```python
from build123d import *

# Parameters (mm, degrees)
F1_DEPTH = 6
F2_R     = 1
F3_R     = 10
F4_DEPTH = 16
F6_DEPTH = 25


with BuildPart() as f1:
    # F0 (on Front) → F1 (new body)
    with BuildSketch(Plane.XZ):
        with BuildLine():
            Line((0.9983844832, 7.6002832444), (-0.5016155168, 7.6002832444))
            ThreePointArc((-0.5016155168, 7.6002832444), (-2.6229358604, 6.7216035879), (-3.5016155168, 4.6002832444))
            Line((-3.5016155168, 4.6002832444), (-3.5016155168, 1.6002832444))
            ThreePointArc((-3.5016155168, 1.6002832444), (-2.6229358604, -0.5210370992), (-0.5016155168, -1.3997167556))
            Line((-0.5016155168, -1.3997167556), (0.9983844832, -1.3997167556))
            ThreePointArc((0.9983844832, -1.3997167556), (3.4732582173, -0.3745904898), (4.4983844832, 2.1002832444))
            Line((4.4983844832, 2.1002832444), (4.4983844832, 4.1002832444))
            ThreePointArc((4.4983844832, 4.1002832444), (3.4732582173, 6.5751569785), (0.9983844832, 7.6002832444))
        make_face()
    extrude(amount=F1_DEPTH)

    # F2
    f2_edges = [f1.edges().sort_by_distance(p)[0] for p in [
        (3.473258, -6, 6.575157),
        (0.248384, -6, 7.600283),
        (-2.622936, -6, 6.721604),
        (-3.501616, -6, 3.100283),
        (-2.622936, -6, -0.521037),
        (0.248384, -6, -1.399717),
        (3.473258, -6, -0.37459),
        (4.498384, -6, 3.100283),
    ]]
    fillet(f2_edges, radius=F2_R)

    # F3 (on face) → F4 (join)
    with BuildSketch(Plane(origin=(0, 0, 0), x_dir=(-1, 0, 0), z_dir=(0, 1, 0))):
        with Locations((-0.2483844832, 3.1002832444)):
            Circle(F3_R)
        with BuildLine():
            Line((3.5016155168, 4.6002832444), (3.5016155168, 3.1002832444))
            Line((3.5016155168, 3.1002832444), (3.5016155168, 1.6002832444))
            ThreePointArc((3.5016155168, 1.6002832444), (2.6229358604, -0.5210370992), (0.5016155168, -1.3997167556))
            Line((0.5016155168, -1.3997167556), (-0.2483844832, -1.3997167556))
            Line((-0.2483844832, -1.3997167556), (-0.9983844832, -1.3997167556))
            ThreePointArc((-0.9983844832, -1.3997167556), (-3.4732582173, -0.3745904898), (-4.4983844832, 2.1002832444))
            Line((-4.4983844832, 2.1002832444), (-4.4983844832, 3.1002832444))
            Line((-4.4983844832, 3.1002832444), (-4.4983844832, 4.1002832444))
            ThreePointArc((-4.4983844832, 4.1002832444), (-3.4732582173, 6.5751569785), (-0.9983844832, 7.6002832444))
            Line((-0.9983844832, 7.6002832444), (-0.2483844832, 7.6002832444))
            Line((-0.2483844832, 7.6002832444), (0.5016155168, 7.6002832444))
            ThreePointArc((0.5016155168, 7.6002832444), (2.6229358604, 6.7216035879), (3.5016155168, 4.6002832444))
        make_face(mode=Mode.SUBTRACT)
        with BuildLine():
            Line((-0.2483844832, -1.3997167556), (-0.2483844832, 3.1002832444))
            Line((-0.2483844832, 3.1002832444), (-4.4983844832, 3.1002832444))
            Line((-4.4983844832, 3.1002832444), (-4.4983844832, 2.1002832444))
            ThreePointArc((-4.4983844832, 2.1002832444), (-3.4732582173, -0.3745904898), (-0.9983844832, -1.3997167556))
            Line((-0.9983844832, -1.3997167556), (-0.2483844832, -1.3997167556))
        make_face()
        with BuildLine():
            Line((-4.4983844832, 3.1002832444), (-0.2483844832, 3.1002832444))
            Line((-0.2483844832, 3.1002832444), (-0.2483844832, 7.6002832444))
            Line((-0.2483844832, 7.6002832444), (-0.9983844832, 7.6002832444))
            ThreePointArc((-0.9983844832, 7.6002832444), (-3.4732582173, 6.5751569785), (-4.4983844832, 4.1002832444))
            Line((-4.4983844832, 4.1002832444), (-4.4983844832, 3.1002832444))
        make_face()
        with BuildLine():
            Line((3.5016155168, 1.6002832444), (3.5016155168, 3.1002832444))
            Line((3.5016155168, 3.1002832444), (-0.2483844832, 3.1002832444))
            Line((-0.2483844832, 3.1002832444), (-0.2483844832, -1.3997167556))
            Line((-0.2483844832, -1.3997167556), (0.5016155168, -1.3997167556))
            ThreePointArc((0.5016155168, -1.3997167556), (2.6229358604, -0.5210370992), (3.5016155168, 1.6002832444))
        make_face()
        with BuildLine():
            Line((-0.2483844832, 3.1002832444), (3.5016155168, 3.1002832444))
            Line((3.5016155168, 3.1002832444), (3.5016155168, 4.6002832444))
            ThreePointArc((3.5016155168, 4.6002832444), (2.6229358604, 6.7216035879), (0.5016155168, 7.6002832444))
            Line((0.5016155168, 7.6002832444), (-0.2483844832, 7.6002832444))
            Line((-0.2483844832, 7.6002832444), (-0.2483844832, 3.1002832444))
        make_face()
    extrude(amount=F4_DEPTH)

    # F5 (on face) → F6 (cut)
    with BuildSketch(Plane.XZ):
        with BuildLine():
            Line((-0.0016155168, 12.6002832444), (0.2483844832, 12.6002832444))
            Line((0.2483844832, 12.6002832444), (0.2483844832, 13.1002832444))
            ThreePointArc((0.2483844832, 13.1002832444), (0.1233747149, 13.0995018417), (-0.0016155168, 13.0971577559))
            Line((-0.0016155168, 13.0971577559), (-0.0016155168, 12.6002832444))
        make_face()
        with BuildLine():
            Line((0.2483844832, 13.1002832444), (0.2483844832, 12.6002832444))
            Line((0.2483844832, 12.6002832444), (0.4983844832, 12.6002832444))
            Line((0.4983844832, 12.6002832444), (0.4983844832, 13.0971577559))
            ThreePointArc((0.4983844832, 13.0971577559), (0.3733942515, 13.0995018417), (0.2483844832, 13.1002832444))
        make_face()
    extrude(amount=-F6_DEPTH, mode=Mode.SUBTRACT)


solid = f1.part
```
For this review, take the finished solid that the model builds, in its own axes (mm). A direction names the side the tool comes from. Give positions to 0.01 mm unless a question says otherwise; leave off trailing zeros. Write each loop counter-clockwise with the first axis right and the second up, starting at its lowest first coordinate (ties: lowest second). Pieces come first, ordered by that corner, then holes.
Item 1: Take a section at C-C (z = 11). Give the boundary of the cut face in (x, y), and give its area (3 significant figures).
Item 2: Take a section at B-B (x = 7.5). Give the boundary of the cut face in (y, z).
Item 3: Wall thickness on probe 1 along Y at (x, z) = (-7, 7.5); probe 2 along Z at (x, y) = (-2.5, 4.5); probe 3 along X at (y, z) = (15.25, 6): over which ranges is each line inside the solid? List them lowest first.
Item 4: Machinability: for faces 1 (the face through (3.5, -2.46, 6.55)), 2 (the face through (0, -2, 7.6)), 3 (the face through (4.498, -2, 3)), which of the approach directions +Z, -Z, +X, -X, +Y, -Y give a long, thin tool a straight path to every point of the face, cutting with its end or side? Answer none if there is none.
Item 5: Take a section at A-A (y = -4.25). Give the boundary of the cut face in (x, z).
Item 6: Insertion check: P1, Ø1.5, axis at x = -4, y = 0.5, coming from the +Z side; P2, Ø1, axis at y = 10, z = -2.5, coming from the -X side; P3, Ø3.5, axis at y = -2, z = 3, coming from the -X side. Each pin has a flat end and moves straight along its axis. Give the tip position at first contact, or say it passes through.
Established:
1. outline: (-5.88, 0) - (6.38, 0) - (6.38, 16) - (-5.88, 16) - close
1. area: 196 mm2
2. outline: (0, -3.79) - (16, -3.79) - (16, 9.99) - (0, 9.99) - close
3. probe 1: y = 0 to 16
3. probe 2: z = -6.51 to 12.72
3. probe 3: x = -9.32 to 9.82
4. face 1: +Z, +X, -Y
4. face 2: +Z, +X, -X, -Y
4. face 3: +Z, -Z, +X, -Y
5. outline: (-3.5, 1.6) arc R3 ccw to (-0.5, -1.4) - (1, -1.4) arc R3.5 ccw to (4.5, 2.1) - (4.5, 4.1) arc R3.5 ccw to (1, 7.6) - (-0.5, 7.6) arc R3 ccw to (-3.5, 4.6) - close
6. P1: stops at z = 12.47
6. P2: stops at x = -8.35
6. P3: stops at x = -3.5
